For this review, take the finished solid that the model builds, in its own axes (mm). Face numbers are marked on the shaded views. A direction names the side the tool comes from. Give positions to 0.01 mm unless a question says otherwise; leave off trailing zeros. Write each loop counter-clockwise with the first axis right and the second up, starting at its lowest first coordinate (ties: lowest second). Pieces come first, ordered by that corner, then holes.
1) For P1, Ø3.5, axis at x = 0, z = 12, coming from the +Y side; P2, Ø12, axis at y = -11, z = 17.5, coming from the +X side; P3, Ø2, axis at x = 14, z = 17.5, coming from the -Y side, all flat-tipped, find the tip position at first contact; note any pin that passes through.
2) Wall thickness on line 1 along Z through (x, y) = (0, 28.5); line 2 along Y through (x, z) = (0, 1.15); line 3 along X through (y, z) = (31, 12): over which ranges is each line inside the solid? List them lowest first.
3) Draft analysis for pull direction Y (two halves, no side actions). For the marked faces 1, 2 and 3, state which applies: pulls with the +Y half, pulls with the -Y half, needs draft (parallel to the pull), parting line crosses it, or undercut.
4) We need section A-A on x = 0. Give the boundary of the cut face in (y, z), and give its area (3 significant figures).
5) We need section B-B on y = 0. Give the boundary of the cut face in (x, z).
6) We need section D-D on x = 12.5. Give the boundary of the cut face in (y, z).
7) We need section C-C on z = 12. Give the boundary of the cut face in (x, y).
8) Machinability: for the marked faces 4, 5 and 6, which of the approach directions +Z, -Z, +X, -X, +Y, -Y give a long, thin tool a straight path to every point of the face, cutting with its end or side? Answer none if there is none.
from build123d import *

# Parameters (mm, degrees)
SKETCH_1_R           = 27
EXTRUDE_1_DEPTH      = 2
SKETCH_2_R           = 27
SKETCH_2_R_2         = 25
EXTRUDE_2_DEPTH      = 30
SKETCH_3_R           = 2.5
CUT_EXTRUDE_1_DEPTH  = 15
EXTRUDE_3_DEPTH      = 10
EXTRUDE_3_DEPTH_BACK = 2
SKETCH_4_R           = 5
SKETCH_5_R           = 3
CUT_EXTRUDE_2_DEPTH  = 50


with BuildPart() as part:
    # 草图1 → 凸台-拉伸1 (new body)
    with BuildSketch(Plane.XY):
        Circle(SKETCH_1_R)
    extrude(amount=EXTRUDE_1_DEPTH)

    # 草图2 → 凸台-拉伸2 (add)
    with BuildSketch(Plane.XY):
        Circle(SKETCH_2_R)
        Circle(SKETCH_2_R_2, mode=Mode.SUBTRACT)
    extrude(amount=EXTRUDE_2_DEPTH)

    # 草图3 → 切除-拉伸1 (cut, symmetric)
    with BuildSketch(Plane.XY):
        Circle(SKETCH_3_R)
    extrude(amount=CUT_EXTRUDE_1_DEPTH, both=True, mode=Mode.SUBTRACT)

    # 草图4 → 凸台-拉伸3 (add, two sides: drawn at the far end of the back side and taken through both)
    with BuildSketch(Plane(origin=(0, 27, 0), x_dir=(1, 0, 0), z_dir=(0, 1, 0)).offset(-EXTRUDE_3_DEPTH_BACK)):
        with Locations(Location((0, -12, 0), (0, 0, 270))):
            Circle(SKETCH_4_R)
    extrude(amount=EXTRUDE_3_DEPTH + EXTRUDE_3_DEPTH_BACK)

    # 草图5 → 切除-拉伸2 (cut)
    with BuildSketch(Plane(origin=(0, 37, 0), x_dir=(1, 0, 0), z_dir=(0, 1, 0))):
        with Locations(Location((0, -12, 0), (0, 0, 270))):
            Circle(SKETCH_5_R)
    extrude(amount=-CUT_EXTRUDE_2_DEPTH, mode=Mode.SUBTRACT)


solid = part.part
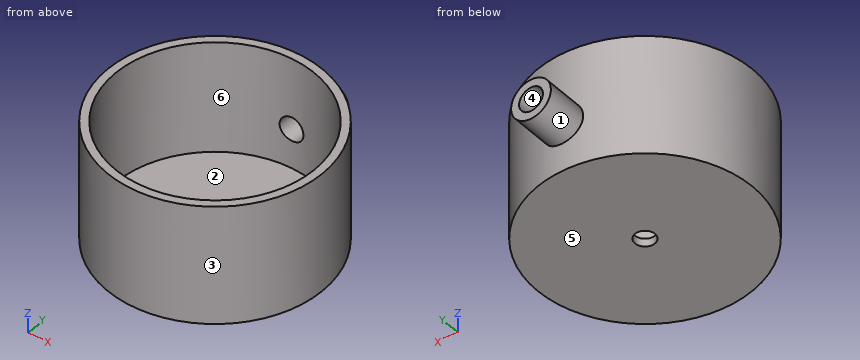
Results list:
1. P1: stops at y = -24.94
1. P2: stops at x = 26.53
1. P3: stops at y = -23.66
2. line 1: z = 7 to 9, 15 to 17
2. line 2: y = -27 to -2.5, 2.5 to 27
2. line 3: x = -5 to -3, 3 to 5
3. face 1: needs draft
3. face 2: undercut
3. face 3: parting line crosses it
4. outline: (-27, 0) - (-2.5, 0) - (-2.5, 2) - (-25, 2) - (-25, 30) - (-27, 30) - close; (2.5, 0) - (27, 0) - (27, 7) - (37, 7) - (37, 9) - (25, 9) - (25, 2) - (2.5, 2) - close; (25, 15) - (37, 15) - (37, 17) - (27, 17) - (27, 30) - (25, 30) - close
4. area: 238 mm2
5. outline: (-27, 0) - (-2.5, 0) - (-2.5, 2) - (-25, 2) - (-25, 30) - (-27, 30) - close; (2.5, 0) - (27, 0) - (27, 30) - (25, 30) - (25, 2) - (2.5, 2) - close
6. outline: (-23.93, 0) - (23.93, 0) - (23.93, 30) - (21.65, 30) - (21.65, 2) - (-21.65, 2) - (-21.65, 30) - (-23.93, 30) - close
7. outline: (-5, 26.53) arc R27 ccw (long way) to (5, 26.53) - (5, 37) - (3, 37) - (3, 24.82) arc R25 cw (long way) to (-3, 24.82) - (-3, 37) - (-5, 37) - close
8. face 4: +Y
8. face 5: -Z, +X, -X, +Y, -Y
8. face 6: +Z
